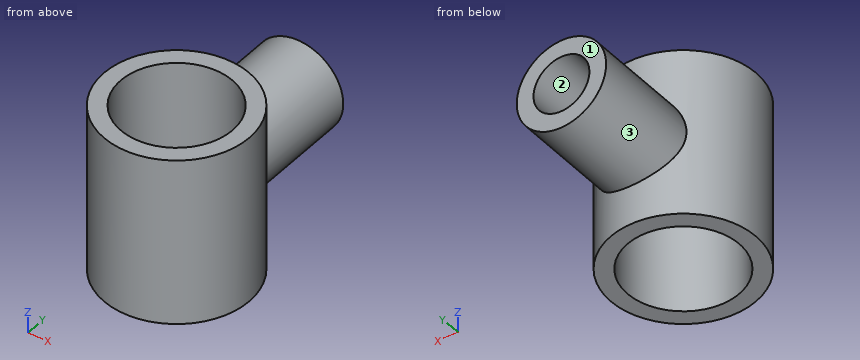
from build123d import *

# Parameters (mm, degrees)
SKETCH1_R           = 4
SKETCH1_R_2         = 2.5
BOSS_EXTRUDE1_DEPTH = 15
SKETCH2_R           = 6.5
BOSS_EXTRUDE3_DEPTH = 7.5
SKETCH3_R           = 5
CUT_EXTRUDE1_DEPTH  = 15


with BuildPart() as part:
    # Sketch1 → Boss-Extrude1 (new body)
    with BuildSketch(Plane(origin=(0, 0, 0), x_dir=(1, 0, 0), z_dir=(0, 1, 0))):
        with Locations(Location((0, 0, 0), (0, 0, 270))):
            Circle(SKETCH1_R)
        with Locations(Location((0, 0, 0), (0, 0, 270))):
            Circle(SKETCH1_R_2, mode=Mode.SUBTRACT)
    extrude(amount=BOSS_EXTRUDE1_DEPTH)

    # Sketch2 → Boss-Extrude3 (add, symmetric)
    with BuildSketch(Plane.XY):
        Circle(SKETCH2_R)
    extrude(amount=BOSS_EXTRUDE3_DEPTH, both=True)

    # Sketch3 → Cut-Extrude1 (cut)
    with BuildSketch(Plane.XY.offset(7.5)):
        Circle(SKETCH3_R)
    extrude(amount=-CUT_EXTRUDE1_DEPTH, mode=Mode.SUBTRACT)


solid = part.part
Source: CAD feature listing. Evaluate the final solid. Frame: model axes, mm. Face numbers are marked on the shaded views. Coordinates: 2 decimals unless noted, no trailing zeros. Loops run counter-clockwise (first coordinate to the right, second up) from the corner with the lowest first, then second, coordinate; pieces in that order, holes last. Notation, with made-up numbers: (-23, 22) - (-9, 22) arc R18 cw to (-9, 27) - close; hole circle Ø11 at (34, 40.25). An arc over 180 degrees is marked (long way). Return JSON: item names as keys, results as strings.
Q1. Section B-B, the plane y = 0. Return loops of the section in (x, z).
Results:
{"outline": "(-6.5, -7.5) - (-5, -7.5) - (-5, 7.5) - (-6.5, 7.5) - close; (5, -7.5) - (6.5, -7.5) - (6.5, 7.5) - (5, 7.5) - close"}
Q2. Contact query for flat-ended pins moving along their axis: P1, Ø1, axis at y = 7, z = -3.5, coming from the -X side; P2, Ø1.5, axis at x = -2.5, y = 13, coming from the +Z side; P3, Ø2, axis at y = 2.5, z = 1, coming from the -X side. Output: stop coordinate, or through.
Results:
{"P1": "x = -2.65", "P2": "z = 3.6", "P3": "x = -6.32"}
Q3. Mould query, pull axis X, two halves, no side actions, for the marked faces 1, 2 and 3. Classes: released by +X, released by -X, zero draft, split by the parting line, or undercut.
Results:
{"face 1": "zero draft", "face 2": "undercut", "face 3": "split by the parting line"}
Q4. Section A-A, the plane x = 0. Return loops of the section in (y, z).
Results:
{"outline": "(-6.5, -7.5) - (-5, -7.5) - (-5, 7.5) - (-6.5, 7.5) - close; (5, -7.5) - (6.5, -7.5) - (6.5, -4) - (15, -4) - (15, -2.5) - (6.5, -2.5) - (6.5, 2.5) - (15, 2.5) - (15, 4) - (6.5, 4) - (6.5, 7.5) - (5, 7.5) - close"}
Q5. Material intervals for line 1 along X through (y, z) = (12.25, 0); line 2 along Y through (x, z) = (0, -2.25), sorted ascending.
Results:
{"line 1": "-4 to -2.5, 2.5 to 4", "line 2": "-6.5 to -5, 5 to 6.5"}
Q6. Section D-D, the plane y = 7.5. Return loops of the section in (x, z), plus the area to 3 significant figures.
Results:
{"outline": "circle Ø8 at (0, 0); hole circle Ø5 at (0, 0)", "area": "30.6 mm2"}
Q7. Section C-C, the plane z = 0. Return loops of the section in (x, y), plus the area to 3 significant figures.
Results:
{"outline": "(-4, 5.12) arc R6.5 ccw (long way) to (4, 5.12) - (4, 15) - (2.5, 15) - (2.5, 6) arc R6.5 ccw to (-2.5, 6) - (-2.5, 15) - (-4, 15) - close; hole circle Ø10 at (0, 0)", "area": "82.4 mm2"}
